Here's how the part is built. I have some questions about the finished solid (model axes, mm). A direction names the side the tool comes from. Round coordinates to 2 decimals unless told otherwise and drop trailing zeros. Loops run counter-clockwise (first coordinate to the right, second up) from the corner with the lowest first, then second, coordinate; pieces in that order, holes last. Notation, with made-up numbers: M 66,61 L 115,61 A22 ccw 115,83 Z; hole C 75.25,8 d7. An arc over 180 degrees is marked long. Use a Markdown table: item, result.
```python
from build123d import *

# Parameters (mm, degrees)
BOSS_EXTRUDE1_DEPTH = 5
SKETCH3_R           = 17.5
SKETCH3_R_2         = 12.5
BOSS_EXTRUDE2_DEPTH = 70


with BuildPart() as part:
    # Sketch1 → Boss-Extrude1 (new body)
    with BuildSketch(Plane(origin=(0, 0, 0), x_dir=(1, 0, 0), z_dir=(0, 1, 0))):
        with BuildLine():
            Line((0, 0), (97.75, 0))
            Line((97.75, 0), (117.746979772, 19.996979772))
            Line((117.746979772, 19.996979772), (117.746979772, 49.996979772))
            Line((117.746979772, 49.996979772), (130.000479502, 49.996979772))
            Line((130.000479502, 49.996979772), (130.000479502, 119.996979772))
            Line((130.000479502, 119.996979772), (117.750479502, 119.996979772))
            Line((117.750479502, 119.996979772), (117.750479502, 139.999520498))
            Line((117.750479502, 139.999520498), (-39.999520498, 139.999520498))
            ThreePointArc((-39.999520498, 139.999520498), (-47.07058831, 137.07058831), (-49.999520498, 129.999520498))
            Line((-49.999520498, 129.999520498), (-49.999520498, 49.999520498))
            Line((-49.999520498, 49.999520498), (0, 0))
        make_face()
    extrude(amount=-BOSS_EXTRUDE1_DEPTH)

    # Sketch3 → Boss-Extrude2 (add)
    with BuildSketch(Plane(origin=(0, 0, -119.996979772), x_dir=(-1, 0, 0), z_dir=(0, 0, -1))):
        with Locations((-129.871326169, -17.499523405)):
            Circle(SKETCH3_R)
        with Locations((-129.871326169, -17.499523405)):
            Circle(SKETCH3_R_2, mode=Mode.SUBTRACT)
    extrude(amount=-BOSS_EXTRUDE2_DEPTH)


solid = part.part
```
Q1. Imagine slicing it at C-C, the plane z = -58. Please give me the cut outline in (x, y), then the cut area to 3 significant figures.
Return value:
| item | result |
|---|---|
| outline | M -50,-5 L 117.62,-5 A17.5 ccw long 129.74,0 L -50,0 Z; hole M 129.76,-5 A12.5 ccw long 129.98,-5 Z |
| area | 1,330 mm^2 |
Q2. For faces 1 (the cylindrical face through (-46.99, -2.46, -137.15)), 2 (the flat face through (117.75, -2, -130)), 3 (the flat face through (117.747, -2, -35)), which set-ups out of +Z, -Z, +X, -X, +Y, -Y let a thin tool reach every point of the face, with its end or its side?
Return value:
| item | result |
|---|---|
| face 1 | -Z, -X, +Y, -Y |
| face 2 | -Z, +X, +Y, -Y |
| face 3 | +Z, +X, +Y, -Y |
Q3. Imagine slicing it at A-A, the plane y = -12.5. Please give me the cut outline in (x, z).
Return value:
| item | result |
|---|---|
| outline | M 113.1,-120 L 118.41,-120 L 118.41,-50 L 113.1,-50 Z; M 141.33,-120 L 146.64,-120 L 146.64,-50 L 141.33,-50 Z |
Q4. Will these pins go through, and if not, where does the flat tip stop? P1, Ø1.5, axis at x = 64.5, z = -124, coming from the -Y side; P2, Ø2.5, axis at y = -3, z = -131, coming from the +X side; P3, Ø1.5, axis at y = -2, z = -28, coming from the +X side.
Return value:
| item | result |
|---|---|
| P1 | stops at y = -5 |
| P2 | stops at x = 117.75 |
| P3 | stops at x = 117.75 |
Q5. Imagine slicing it at D-D, the plane z = -27. Please give me the cut outline in (x, y), then the cut area to 3 significant figures.
Return value:
| item | result |
|---|---|
| outline | M -27,-5 L 117.75,-5 L 117.75,0 L -27,0 Z |
| area | 724 mm^2 |
Q6. I need wall thicknesses on line 1 (Y direction, x = 19, z = -27); line 2 (Y direction, x = 136.5, z = -51.5); line 3 (X direction, y = -13, z = -58.5). Which ranges of each line are inside material? Lowest first, please. Write a range as from..to.
Return value:
| item | result |
|---|---|
| line 1 | y = -5..0 |
| line 2 | y = -33.7..-28.1, -6.9..-1.3 |
| line 3 | x = 112.96..118.21, 141.53..146.78 |
Q7. Imagine slicing it at B-B, the plane x = 123. Please give me the cut outline in (y, z).
Return value:
| item | result |
|---|---|
| outline | M -33.59,-120 L -27.94,-120 L -27.94,-50 L -33.59,-50 Z; M -7.06,-120 L 0,-120 L 0,-50 L -7.06,-50 Z |
